from build123d import *

# Parameters (mm, degrees)
F0_W     = 16
F0_H     = 2.4
F0_W_2   = 348
F0_H_2   = 1.2
F2_R     = 2
F3_DEPTH = 15
F4_W     = 10
F4_H     = 0.5
F5_DEPTH = 10
F6_R     = 0.775
F7_DEPTH = 340


with BuildPart() as f1:
    # F0 (on Front) → F1 (revolve)
    with BuildSketch(Plane.XZ):
        with Locations((18.878411, 1.2)):
            Rectangle(F0_W, F0_H)
        Polygon((-8.121589, 0), (10.878411, 0), (10.878411, 2.4), (-8.121589, 1.2), align=None)
        with Locations((-182.121589, 0.6)):
            Rectangle(F0_W_2, F0_H_2)
    revolve(axis=Axis((11.143533, 0, 0), (1, 0, 0)))

    # F2 (on face) → F3 (cut)
    with BuildSketch(Plane.YZ.offset(26.878411)):
        Circle(F2_R)
    extrude(amount=-F3_DEPTH, mode=Mode.SUBTRACT)

    # F4 (on Front) → F5 (cut)
    with BuildSketch(Plane.XZ):
        with Locations((21.878411, 0)):
            Rectangle(F4_W, F4_H)
    extrude(amount=F5_DEPTH, mode=Mode.SUBTRACT)

    # F6 (on face) → F7 (cut)
    with BuildSketch(Plane(origin=(-356.121589, 0, 0), x_dir=(0, -1, 0), z_dir=(-1, 0, 0))):
        Circle(F6_R)
    extrude(amount=-F7_DEPTH, mode=Mode.SUBTRACT)


solid = f1.part
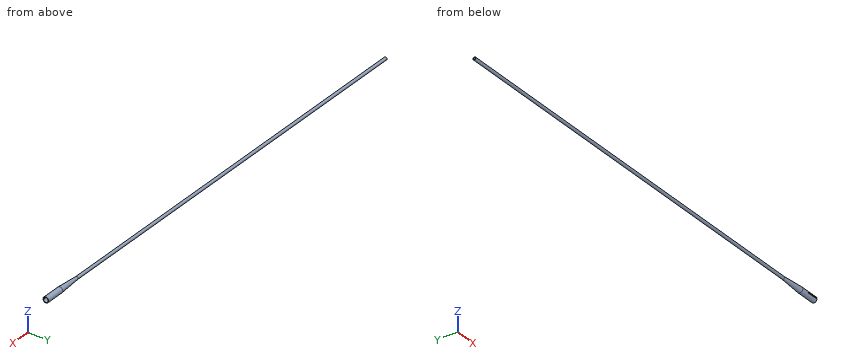
Check sheet for the modelled part. Datum: model origin and axes. Units: mm. Round coordinates to 2 decimals unless told otherwise and drop trailing zeros. Order: outer loops, then holes, each group sorted by start corner. A loop starts at its lowest first (then second) coordinate and runs counter-clockwise, first axis right, second up.
(1) Cross-section at B-B, the plane x = -282.5. Enter the section's corners in (y, z) (3 decimals), and give its area (3 significant figures).
(2) Cross-section at A-A, the plane y = 0. Enter the section's corners in (x, z) (3 decimals).
(3) Scan lines: probe 1 along Z at (x, y) = (-122.5, -0.05); probe 2 along Z at (x, y) = (23, 0); probe 3 along X at (y, z) = (-0.35, 0). Record each from-to range of solid material in increasing order.
(4) Go/stop test with flat-tipped pins: P1, Ø2.5, axis at y = 0, z = 0, coming from the +X side; P2, Ø2, axis at x = -269, z = -1.5, coming from the +Y side; P3, Ø1.5, axis at x = -181.5, z = -0.5, coming from the +Y side. Record where each tip stops, or that it passes through.
Check sheet entries:
1. outline: circle Ø2.4 at (0, 0); hole circle Ø1.55 at (0, 0)
1. area: 2.64 mm2
2. outline: (-356.122, -1.2) - (-8.122, -1.2) - (10.878, -2.4) - (26.878, -2.4) - (26.878, -2) - (11.878, -2) - (11.878, 2) - (26.878, 2) - (26.878, 2.4) - (10.878, 2.4) - (-8.122, 1.2) - (-356.122, 1.2) - (-356.122, 0.775) - (-16.122, 0.775) - (-16.122, -0.775) - (-356.122, -0.775) - close
3. probe 1: z = -1.2 to -0.77, 0.77 to 1.2
3. probe 2: z = -2.4 to -2, 2 to 2.4
3. probe 3: x = -16.12 to 11.88
4. P1: stops at x = 11.88
4. P2: stops at y = 1.09
4. P3: stops at y = 1.2
